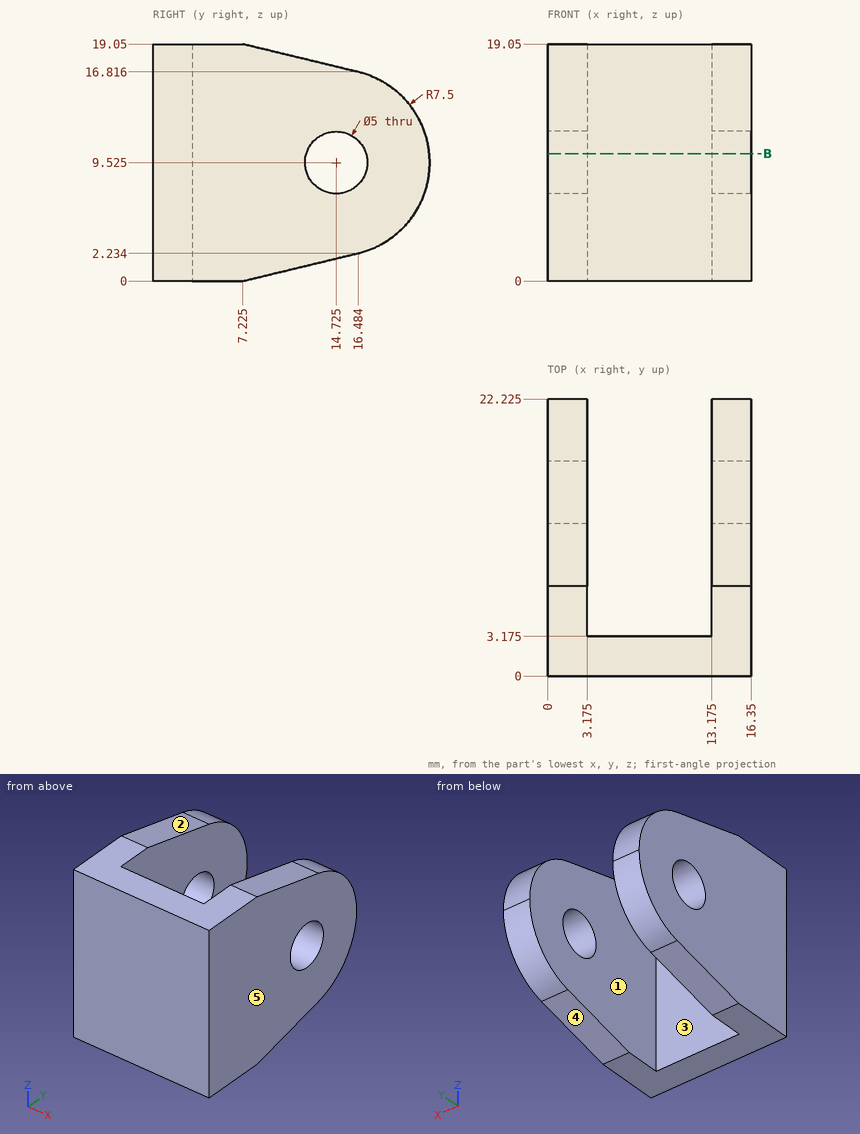
Verification items for this drawing (mm, ordinates from the low corner). A direction names the side the tool comes from. Give positions to 0.01 mm unless a question says otherwise; leave off trailing zeros. Answer as a JSON object with one key per item and string values. Group by question number.
Item 1: Access from +Z, -Z, +X, -X, +Y, -Y to the whole of each face (thin tool, end or side, straight path). Record for the marked faces 1 and 2.
Item 2: Material ranges on L1, parallel to Y at x = 3, z = 8.25 (1 decimal); L2, parallel to Y at x = 10.75, z = 7.75 (1 decimal); L3, parallel to Y at x = 1.5, z = 12.75, recorded low to high.
Item 3: Gauge pin test, flat ends, axial feed: pin 1 (1.5 mm diameter, centred on x = 13.5, z = 11, fed in from +Y); pin 2 (1.5 mm diameter, centred on x = 5, z = 16, fed in from +Y) (3 decimals); pin 3 (3 mm diameter, centred on y = 14.725, z = 9.525, fed in from +X); pin 4 (4 mm diameter, centred on x = 11.5, y = 10.5, fed in from -Z). Record the tip position at first contact, or that the pin passes through.
Item 4: Sectioned sample at B-B on z = 10.25. Give the number of separate pieces and of enclosed holes in the cut face, plus the area to 3 significant figures.
Item 5: Mould release check, pull along X, two halves, no side actions. Record for the marked faces 3, 4 and 5: pulls with the +X half, pulls with the -X half, needs draft (parallel to the pull), parting line crosses it, or undercut.
Findings below:
{
 "1": {"face 1": "+Z, -Z, +Y", "face 2": "+Z, +X, -X, +Y"},
 "2": {"L1": "0 to 12.6, 16.9 to 22.1", "L2": "0 to 3.2", "L3": "0 to 21.5"},
 "3": {"pin 1": "y = 22.19", "pin 2": "y = 3.175", "pin 3": "through", "pin 4": "z = 0.53"},
 "4": {"separate pieces": "3", "enclosed holes": "0", "area": "142 mm2"},
 "5": {"face 3": "undercut", "face 4": "needs draft", "face 5": "pulls with the +X half"}
}
